```python
from build123d import *

# Parameters (mm, degrees)
BOSS_EXTRUDE1_DEPTH = 1
SKETCH2_R           = 3.5
BOSS_EXTRUDE2_DEPTH = 3.5
SKETCH3_R           = 1.25
BOSS_EXTRUDE3_DEPTH = 3


with BuildPart() as part:
    # Sketch1 → Boss-Extrude1 (new body)
    with BuildSketch(Plane.XY):
        Polygon((-61.85, 33.5), (-61.85, 21.8), (-51.85, 21.8), (-51.85, -32.2), (-61.85, -32.2), (-61.85, -33.5), (62.65, -33.5), (62.65, 33.5), align=None)
    extrude(amount=BOSS_EXTRUDE1_DEPTH)

    # Sketch2 → Boss-Extrude2 (add)
    with BuildSketch(Plane.XY.offset(1)):
        with Locations(Location((-24.25, 24.5, 0), (0, 0, 180))):
            Circle(SKETCH2_R)
        with Locations(Location((33.75, 24.5, 0), (0, 0, 180))):
            Circle(SKETCH2_R)
        with Locations(Location((33.75, -24.5, 0), (0, 0, 180))):
            Circle(SKETCH2_R)
        with Locations(Location((-24.25, -24.5, 0), (0, 0, 180))):
            Circle(SKETCH2_R)
    extrude(amount=BOSS_EXTRUDE2_DEPTH)

    # Sketch3 → Boss-Extrude3 (add)
    with BuildSketch(Plane.XY.offset(4.5)):
        with Locations((-24.25, 24.5)):
            Circle(SKETCH3_R)
        with Locations((33.75, 24.5)):
            Circle(SKETCH3_R)
        with Locations((33.75, -24.5)):
            Circle(SKETCH3_R)
        with Locations((-24.25, -24.5)):
            Circle(SKETCH3_R)
    extrude(amount=BOSS_EXTRUDE3_DEPTH)


solid = part.part
```
Can you work these out from the model? Positions are in its coordinate system, mm. A direction names the side the tool comes from. Coordinates: 2 decimals unless noted, no trailing zeros. Order: outer loops, then holes, each group sorted by start corner. A loop starts at its lowest first (then second) coordinate and runs counter-clockwise, first axis right, second up. Notation, with made-up numbers: (20, 20) -> (55, 20) arc R10 cw to (55, 25) -> close; hole circle Ø7 at (5, 5.5). An arc over 180 degrees is marked (long way). Write each question's results on one line, items separated by ' | '.
Item 1: I want a section at D-D, the plane y = 11. Write out the boundary of the cut face in (x, z).
Results are:
outline: (-51.85, 0) -> (62.65, 0) -> (62.65, 1) -> (-51.85, 1) -> close
Item 2: I want a section at A-A, the plane y = 24.5. Write out the boundary of the cut face in (x, z), then the cut area to 4 significant figures.
Results are:
outline: (-61.85, 0) -> (62.65, 0) -> (62.65, 1) -> (37.25, 1) -> (37.25, 4.5) -> (35, 4.5) -> (35, 7.5) -> (32.5, 7.5) -> (32.5, 4.5) -> (30.25, 4.5) -> (30.25, 1) -> (-20.75, 1) -> (-20.75, 4.5) -> (-23, 4.5) -> (-23, 7.5) -> (-25.5, 7.5) -> (-25.5, 4.5) -> (-27.75, 4.5) -> (-27.75, 1) -> (-61.85, 1) -> close | area: 188.5 mm²
Item 3: I want a section at B-B, the plane z = 2.25. Write out the boundary of the cut face in (x, y).
Results are:
outline: circle Ø7 at (-24.25, -24.5); circle Ø7 at (-24.25, 24.5); circle Ø7 at (33.75, -24.5); circle Ø7 at (33.75, 24.5)
Item 4: If we mould it in two halves opening along X, with no side actions, what happens to faces 3 (the face through (-24, 26, 4.5)), 4 (the face through (-26.13, -27.45, 2.73)), 5 (the face through (-24, -24, 7.5))? For each: +X half, -X half, draft (parallel to the pull), parting line (faces both ways), or undercut.
Results are:
face 3: undercut | face 4: undercut | face 5: draft
Item 5: Which directions (+Z, -Z, +X, -X, +Y, -Y) give clear straight access to the entire face, cutting with the end or side of a thin tool? Please do faces 1 (the face through (0, 0, 0)), 2 (the face through (34, 26, 4.5)).
Results are:
face 1: -Z, +X, -X, +Y, -Y | face 2: +Z
Item 6: I want a section at C-C, the plane x = -24.25. Write out the boundary of the cut face in (y, z).
Results are:
outline: (-33.5, 0) -> (33.5, 0) -> (33.5, 1) -> (28, 1) -> (28, 4.5) -> (25.75, 4.5) -> (25.75, 7.5) -> (23.25, 7.5) -> (23.25, 4.5) -> (21, 4.5) -> (21, 1) -> (-21, 1) -> (-21, 4.5) -> (-23.25, 4.5) -> (-23.25, 7.5) -> (-25.75, 7.5) -> (-25.75, 4.5) -> (-28, 4.5) -> (-28, 1) -> (-33.5, 1) -> close
Item 7: If I drill on line 1 along Z through (x, y) = (39, -15); line 2 along Z through (x, y) = (-24, 26); line 3 along X through (y, z) = (-23, 3.25), over which ranges is the centre line in solid material (lowest first)?
Results are:
line 1: 0 to 1 | line 2: 0 to 4.5 | line 3: -27.41 to -21.09, 30.59 to 36.91
Item 8: I'm going to push flat-ended pins straight in: pin 1 Ø3 at (y, z) = (-3.5, 2) entering from -X; pin 2 Ø6 at (x, y) = (-20, 13) entering from +Z. Where does each tip first touch, or does it pass through?
Results are:
pin 1: x = -51.85 | pin 2: z = 1
